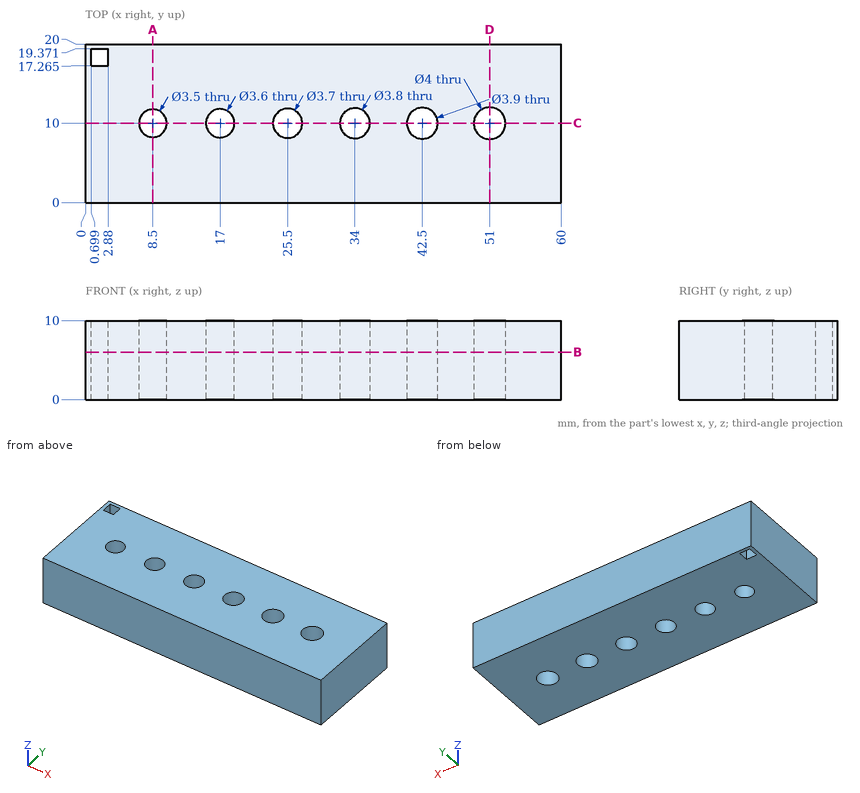
Verification items for this drawing (mm, ordinates from the low corner). Coordinates: 2 decimals unless noted, no trailing zeros. Order: outer loops, then holes, each group sorted by start corner. A loop starts at its lowest first (then second) coordinate and runs counter-clockwise, first axis right, second up. Notation, with made-up numbers: M -8,-12 L 46,-12 A25 ccw 46,9 Z; hole C -0.75,12 d6. An arc over 180 degrees is marked long. Answer as a JSON object with one key per item and string values.
Q1. Cross-section at D-D on x = 51. Record the cut outline in (y, z).
Results are:
{"outline": "M 0,0 L 8,0 L 8,10 L 0,10 Z; M 12,0 L 20,0 L 20,10 L 12,10 Z"}
Q2. Cross-section at C-C on y = 10. Record the cut outline in (x, z), and give its area (3 significant figures).
Results are:
{"outline": "M 0,0 L 6.75,0 L 6.75,10 L 0,10 Z; M 10.25,0 L 15.2,0 L 15.2,10 L 10.25,10 Z; M 18.8,0 L 23.65,0 L 23.65,10 L 18.8,10 Z; M 27.35,0 L 32.1,0 L 32.1,10 L 27.35,10 Z; M 35.9,0 L 40.55,0 L 40.55,10 L 35.9,10 Z; M 44.45,0 L 49,0 L 49,10 L 44.45,10 Z; M 53,0 L 60,0 L 60,10 L 53,10 Z", "area": "375 mm²"}
Q3. Scan lines: line 1 (Y direction, x = 42.5, z = 7); line 2 (Y direction, x = 8.5, z = 2.5). Record each from-to range of solid material in increasing order.
Results are:
{"line 1": "y = 0 to 8.05, 11.95 to 20", "line 2": "y = 0 to 8.25, 11.75 to 20"}
Q4. Depth check by flat-ended pin: pin 1 Ø1 at (x, y) = (39, 14) entering from -Z. Enter the tip coordinate at first touch or a pass-through.
Results are:
{"pin 1": "stops at z = 0"}
Q5. Cross-section at A-A on x = 8.5. Record the cut outline in (y, z), and give its area (3 significant figures).
Results are:
{"outline": "M 0,0 L 8.25,0 L 8.25,10 L 0,10 Z; M 11.75,0 L 20,0 L 20,10 L 11.75,10 Z", "area": "165 mm²"}
Q6. Cross-section at B-B on z = 6. Give the number of separate pieces and of enclosed holes in the cut face, and give its area (3 significant figures).
Results are:
{"separate pieces": "1", "enclosed holes": "7", "area": "1,130 mm²"}
